Design review of the part built by this model. Coordinates are the model's own, in mm. A direction names the side the tool comes from. Round coordinates to 2 decimals unless told otherwise and drop trailing zeros. Loops run counter-clockwise (first coordinate to the right, second up) from the corner with the lowest first, then second, coordinate; pieces in that order, holes last. Notation, with made-up numbers: (-8, -16) -> (-2, -16) arc R20 ccw to (-2, 4) -> close; hole circle Ø3 at (-38, 61). An arc over 180 degrees is marked (long way). Answer as CSV lines item,"result". Start each with the question number.
(1) For P1, Ø1.8, axis at x = 62.91, y = 21.53, coming from the -Z side; P2, Ø0.9, axis at x = -55, z = 2.5, coming from the -Y side; P3, Ø1, axis at y = 5.5, z = 2, coming from the -X side; P4, Ø2, axis at y = -5, z = 2, coming from the +X side, all flat-tipped, find the tip position at first contact; note any pin that passes through.
(2) Take a section at B-B, the plane z = 1.35. State how many separate pieces and enclosed holes the cut face has, and give its area (3 significant figures).
(3) Machinability: for faces 1 (the face through (-15.094, -4, 2)), 2 (the face through (60.906, -4, 2)), 3 (the face through (3, 19, 3.5)), 4 (the face through (-54.094, -4, 2)), which of the approach directions +Z, -Z, +X, -X, +Y, -Y give a long, thin tool a straight path to every point of the face, cutting with its end or side? Answer none if there is none.
(4) To check wall thickness, follow line 1 (X direction, y = -18, z = 0.45); line 2 (Y direction, x = -29, z = 2.9); line 3 (Y direction, x = -37, z = 3). State the ranges of each line that lie inside material, in increasing order. Write a range as from..to.
(5) Draft analysis for pull direction X (two halves, no side actions). For faces 5 (the face through (-69.094, 22, 2)), 6 (the face through (26, -22.428, 2)), 7 (the face through (75.906, 21, 2)), 8 (the face through (-46.094, -4, 2)), state which applies: +X half, -X half, draft (parallel to the pull), parting line (faces both ways), or undercut.
(6) Take a section at C-C, the plane x = 13. Write out the cut boundary in (y, z).
(7) Take a section at A-A, the plane y = -4.5. Write out the cut boundary in (x, z).
from build123d import *

# Parameters (mm, degrees)
F0_W     = 2.9513968527
F0_H     = 5.7922647223
F0_W_2   = 10.2618969977
F0_H_2   = 6.2077352777
F0_W_3   = 16.8588273227
F0_W_4   = 37.1382929152
F0_W_5   = 8
F0_H_3   = 38
F0_W_6   = 8.1014430672
F0_W_7   = 8.0087523311
F0_W_8   = 8.027805835
F1_DEPTH = 3.5
F2_D     = 2
F3_D     = 3


# Not quite as in the source:
# - a feature names something its author has since deleted; it is built from what else it names


with BuildPart() as f1:
    # F0 (on Top) → F1 (new body)
    with BuildSketch(Plane.XY):
        with Locations((-67.6180190593, 24.675444182)):
            Rectangle(F0_W, F0_H)
        with Locations((-61.0113721341, 24.675444182)):
            Rectangle(F0_W_2, F0_H)
        with Locations((-67.6180190593, 18.675444182)):
            Rectangle(F0_W, F0_H_2)
        with Locations((-47.4510099739, 24.675444182)):
            Rectangle(F0_W_3, F0_H)
        with Locations((-61.0113721341, 18.675444182)):
            Rectangle(F0_W_2, F0_H_2)
        with Locations((-20.4524498549, 24.675444182)):
            Rectangle(F0_W_4, F0_H)
        Polygon((-39.0215963125, 21.7793118209), (-55.8804236352, 21.7793118209), (-55.8804236352, 15.5715765432), (-54.0937174857, 15.5715765432), (-46.0937174857, 15.5715765432), (-39.0215963125, 15.5715765432), align=None)
        Polygon((9.8445750773, 27.5715765432), (-1.8833033973, 27.5715765432), (-1.8833033973, 21.7793118209), (9.8743605615, 21.7793118209), align=None)
        Polygon((-1.8833033973, 21.7793118209), (-39.0215963125, 21.7793118209), (-39.0215963125, 15.5715765432), (-23.1951605529, 15.5715765432), (-15.0937174857, 15.5715765432), (-1.8833033973, 15.5715765432), align=None)
        Polygon((62.8643706441, 27.5715765432), (9.8445750773, 27.5715765432), (9.8743605615, 21.7793118209), (62.8643706441, 21.7793118209), align=None)
        Polygon((9.8743605615, 21.7793118209), (-1.8833033973, 21.7793118209), (-1.8833033973, 15.5715765432), (9.9062825143, 15.5715765432), align=None)
        with Locations((-50.0937174857, -3.4284234568)):
            Rectangle(F0_W_5, F0_H_3)
        Polygon((72.6376026869, 27.5715765432), (62.8643706441, 27.5715765432), (62.8643706441, 21.7793118209), (72.7672914107, 21.7793118209), align=None)
        Polygon((62.8643706441, 21.7793118209), (9.8743605615, 21.7793118209), (9.9062825143, 15.5715765432), (21.8975301832, 15.5715765432), (29.9062825143, 15.5715765432), (52.8784766793, 15.5715765432), (60.9062825143, 15.5715765432), (62.8643706441, 15.5715765432), align=None)
        with Locations((-19.1444390193, -3.4284234568)):
            Rectangle(F0_W_6, F0_H_3)
        Polygon((75.9062825143, 27.5715765432), (72.6376026869, 27.5715765432), (72.7672914107, 21.7793118209), (75.9062825143, 21.7793118209), align=None)
        Polygon((72.7672914107, 21.7793118209), (62.8643706441, 21.7793118209), (62.8643706441, 15.5715765432), (72.9062825143, 15.5715765432), align=None)
        Polygon((75.9062825143, 21.7793118209), (72.7672914107, 21.7793118209), (72.9062825143, 15.5715765432), (75.9062825143, 15.5715765432), align=None)
        with Locations((25.9019063488, -3.4284234568)):
            Rectangle(F0_W_7, F0_H_3)
        with Locations((56.8923795968, -3.4284234568)):
            Rectangle(F0_W_8, F0_H_3)
    extrude(amount=F1_DEPTH)

    # F2 (through all)
    with Locations(Plane(origin=(0, 0, 0), x_dir=(1, 0, 0), z_dir=(0, 0, -1))):
        with Locations((-66.0937174857, -21.7793118209), (-56.0937174857, -21.7793118209), (-39.0937174857, -21.7793118209), (-19.0937174857, -21.7793118209), (-2.0937174857, -21.7793118209), (9.9062825143, -21.7793118209), (25.9062825143, -21.7793118209), (45.9062825143, -21.7793118209), (62.9062825143, -21.5349812061), (72.9062825143, -21.5349812061)):
            Hole(F2_D / 2)

    # F3 (through all)
    with Locations(Plane(origin=(0, 0, 0), x_dir=(1, 0, 0), z_dir=(0, 0, -1))):
        with Locations((-29.0937174857, -21.7793118209), (35.9062825143, -21.7793118209)):
            Hole(F3_D / 2)


solid = f1.part
The answers:
1,P1,"through"
1,P2,"y = 15.57"
1,P3,"x = -54.09"
1,P4,"x = 60.91"
2,separate pieces,"1"
2,enclosed holes,"12"
2,area,"2,920 mm²"
3,face 1,"+Z, -Z, -Y"
3,face 2,"+Z, -Z, +X, -Y"
3,face 3,"+Z, +X, -X, +Y, -Y"
3,face 4,"+Z, -Z, -X, -Y"
4,line 1,"-54.09..-46.09, -23.2..-15.09, 21.9..29.91, 52.88..60.91"
4,line 2,"15.57..20.28, 23.28..27.57"
4,line 3,"15.57..27.57"
5,face 5,"-X half"
5,face 6,"draft"
5,face 7,"+X half"
5,face 8,"undercut"
6,outline,"(15.57, 0) -> (27.57, 0) -> (27.57, 3.5) -> (15.57, 3.5) -> close"
7,outline,"(-54.09, 0) -> (-46.09, 0) -> (-46.09, 3.5) -> (-54.09, 3.5) -> close; (-23.2, 0) -> (-15.09, 0) -> (-15.09, 3.5) -> (-23.2, 3.5) -> close; (21.9, 0) -> (29.91, 0) -> (29.91, 3.5) -> (21.9, 3.5) -> close; (52.88, 0) -> (60.91, 0) -> (60.91, 3.5) -> (52.88, 3.5) -> close"
